Input: part model. Units: mm. Frame: model coordinates. Give positions to 0.01 mm unless a question says otherwise; leave off trailing zeros. Write each loop counter-clockwise with the first axis right and the second up, starting at its lowest first coordinate (ties: lowest second). Pieces come first, ordered by that corner, then holes. Notation, with made-up numbers: (19.25, 88) -> (68.25, 88) arc R38 ccw to (68.25, 126) -> close; hole circle Ø4 at (-3.5, 9). An arc over 180 degrees is marked (long way). Return JSON: item names as keys, results as strings. Group by question number.
Item 1: Section C-C, the plane y = 0.2. Count the separate pieces of the cut face and the enclosed holes in it, then the cut area to 3 significant figures.
Item 2: Section A-A, the plane x = -10.5. Return loops of the section in (y, z).
Item 3: Section B-B, the plane z = -20. Return loops of the section in (x, y), then the cut area to 3 significant figures.
Item 4: Line query: line 1 (Z direction, x = 32, y = 0.7); line 2 (X direction, y = 0.6, z = -8); line 3 (X direction, y = 0.4, z = -7.5). Output: solid intervals per line, ascending. Write a range as [from, to].
Item 5: Pin query (flat end, axial travel): P1, Ø1.7, axis at x = 32, z = -8, coming from the -Y side. Return the tip coordinate at first contact, or that it passes through.
Item 6: Section D-D, the plane x = -24. Return loops of the section in (y, z), then the cut area to 3 significant figures.
from build123d import *

# Parameters (mm, degrees)
BOSS_EXTRUDE2_DEPTH        = 1
FILLET1_R                  = 1
FILLET2_R                  = 0.5
M2_5_CLEARANCE_HOLE1_D     = 2.9
M2_5_CLEARANCE_HOLE1_DEPTH = 7.25
M2_5_CLEARANCE_HOLE1_TIP   = 0.871247898


with BuildPart() as part:
    # Sketch6 → Boss-Extrude2 (new body)
    with BuildSketch(Plane(origin=(0, 0, 0), x_dir=(1, 0, 0), z_dir=(0, 1, 0))):
        Polygon((-21.18242301, -23.733545037), (-14, -4), (-14, -24), (32, -24), (49.571034579, -5.897463907), (40, -3), (15, 0), (40, 3), (49.571034579, 5.897463907), (32, 24), (-14, 24), (-14, 4), (-21.18242301, 23.733545037), (-37.579939109, 14.722767652), (-38.229006165, 8.757978304), (-42.181953388, 4.244198486), (-46.02292771, 5.360852532), (-47, 2), (-45, 2), (-45, -2), (-47, -2), (-46.02292771, -5.360852532), (-42.181953388, -4.244198486), (-38.229006165, -8.757978304), (-37.579939109, -14.722767652), align=None)
        with BuildLine():
            Line((-7, 0), (-13.002008181, -2.57228922))
            ThreePointArc((-13.002008181, -2.57228922), (-12.400581568, 0), (-13.002008181, 2.57228922))
            Line((-13.002008181, 2.57228922), (-7, 0))
        make_face(mode=Mode.SUBTRACT)
    extrude(amount=BOSS_EXTRUDE2_DEPTH)

    # Fillet1
    fillet1_edges = [part.edges().sort_by_distance(p)[0] for p in [
        (-14, 0.5, -24),
        (32, 0.5, -24),
        (49.571034579, 0.5, -5.897463907),
        (40, 0.5, -3),
        (40, 0.5, 3),
        (49.571034579, 0.5, 5.897463907),
        (32, 0.5, 24),
        (-14, 0.5, 24),
        (-21.18242301, 0.5, 23.733545037),
        (-37.579939109, 0.5, 14.722767652),
        (-38.229006165, 0.5, 8.757978304),
        (-42.181953388, 0.5, 4.244198486),
        (-46.02292771, 0.5, 5.360852532),
        (-45, 0.5, 2),
        (-21.18242301, 0.5, -23.733545037),
        (-37.579939109, 0.5, -14.722767652),
        (-38.229006165, 0.5, -8.757978304),
        (-42.181953388, 0.5, -4.244198486),
        (-46.02292771, 0.5, -5.360852532),
        (-45, 0.5, -2),
    ]]
    fillet(fillet1_edges, radius=FILLET1_R)

    # Fillet2
    fillet2_edges = [part.edges().sort_by_distance(p)[0] for p in [
        (-7, 0.5, 0),
        (-13.002008181, 0.5, -2.57228922),
        (-14, 0.5, -4),
        (15, 0.5, 0),
        (-14, 0.5, 4),
        (-13.002008181, 0.5, 2.57228922),
    ]]
    fillet(fillet2_edges, radius=FILLET2_R)

    # M2.5 Clearance Hole1
    with Locations(Plane(origin=(0, 1, 0), x_dir=(1, 0, 0), z_dir=(0, 1, 0))):
        with Locations((-32, 0), (32, 8), (32, -8)):
            Hole(M2_5_CLEARANCE_HOLE1_D / 2, depth=M2_5_CLEARANCE_HOLE1_DEPTH)
            with Locations((0, 0, -(M2_5_CLEARANCE_HOLE1_DEPTH + M2_5_CLEARANCE_HOLE1_TIP / 2))):  # 118° drill point
                Cone(0, M2_5_CLEARANCE_HOLE1_D / 2, M2_5_CLEARANCE_HOLE1_TIP, mode=Mode.SUBTRACT)


solid = part.part
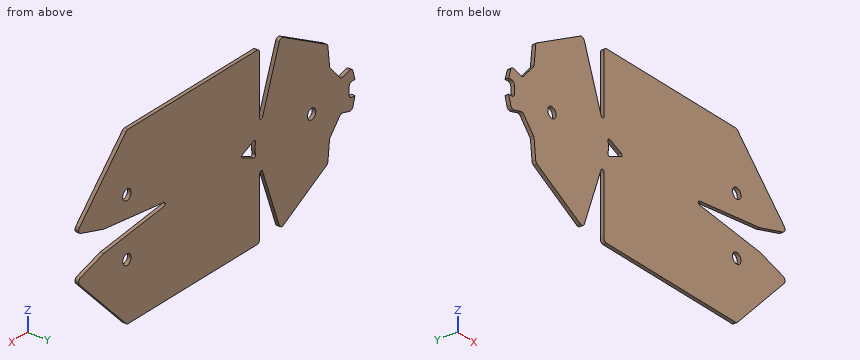
Answer below:
{
 "1": {"separate pieces": "1", "enclosed holes": "4", "area": "3,470 mm2"},
 "2": {"outline": "(0, -24) -> (1, -24) -> (1, -1.5) -> (0, -1.5) -> close; (0, 1.5) -> (1, 1.5) -> (1, 24) -> (0, 24) -> close"},
 "3": {"outline": "(-27.98, 0) -> (-19.82, 0) -> (-19.82, 1) -> (-27.98, 1) -> close; (-14, 0) -> (35.88, 0) -> (35.88, 1) -> (-14, 1) -> close", "area": "58.0 mm2"},
 "4": {"line 1": "z = [-23.91, -9.45], [-6.55, -2.04], [2.04, 6.55], [9.45, 23.91]", "line 2": "x = [-38.89, -15.46], [-14, 30.55], [33.45, 47.53]", "line 3": "x = [-39.33, -15.27], [-14, 30.64], [33.36, 48.02]"},
 "5": {"P1": "passes through"},
 "6": {"outline": "(0, -22.19) -> (1, -22.19) -> (1, 22.19) -> (0, 22.19) -> close", "area": "44.4 mm2"}
}
